Geometry check sheet. Reference: the model listing, model coordinates, mm. A direction names the side the tool comes from. Round coordinates to 2 decimals unless told otherwise and drop trailing zeros. Order: outer loops, then holes, each group sorted by start corner. A loop starts at its lowest first (then second) coordinate and runs counter-clockwise, first axis right, second up.
(1) Set-up check for faces 4 (the face through (11, 0, 12.7)), 5 (the face through (-8, -7, 7.62)): record each of +Z, -Z, +X, -X, +Y, -Y from which the full face is reachable in a straight line by a thin tool's end or side.
(2) Draft check along Y on faces 1 (the face through (-3.472, 26.443, 7.549)), 2 (the face through (13, -24, 2.54)), 3 (the face through (10.902, 3.433, 3.757)). Enter one of: pulls with the +Y half, pulls with the -Y half, needs draft (parallel to the pull), parting line crosses it, or undercut.
(3) Cross-section at A-A on y = 0. Enter the section's corners in (x, z), and give its area (3 significant figures).
(4) Cross-section at C-C on z = 11.25. Enter the section's corners in (x, y).
(5) Cross-section at D-D on x = 21. Enter the section's corners in (y, z).
(6) Thickness scan on L1, parallel to Y at x = 0, z = 3; L2, parallel to Y at x = 0, z = 2.5; L3, parallel to X at y = 0, z = 10.2. Record the ranges inside material, lowest first.
(7) Gauge pin test, flat ends, axial feed: P1, Ø5, axis at y = -22, z = 2.5, coming from the -X side; P2, Ø17.5, axis at x = -1, y = -4, coming from the +Z side; P3, Ø3, axis at y = -11, z = 6, coming from the +X side; P4, Ø20.5, axis at x = 0, y = 0, coming from the -Z side. Record the tip position at first contact, or that the pin passes through.
from build123d import *

# Parameters (mm, degrees)
F0_R     = 29.21
F1_DEPTH = 2.54
F2_R     = 26.67
F3_DEPTH = 12.7
F4_R     = 10.16
F5_DEPTH = 12.701
F6_R     = 11.43
F7_DEPTH = 7.62


with BuildPart() as f1:
    # F0 (on Top) → F1 (new body)
    with BuildSketch(Plane.XY):
        Circle(F0_R)
    extrude(amount=F1_DEPTH)

    # F2 (on Top) → F3 (join)
    with BuildSketch(Plane.XY):
        Circle(F2_R)
    extrude(amount=F3_DEPTH)

    # F4 (on Top) → F5 (cut, through all)
    with BuildSketch(Plane.XY):
        Circle(F4_R)
    extrude(amount=F5_DEPTH, mode=Mode.SUBTRACT)

    # F6 (on Top) → F7 (cut)
    with BuildSketch(Plane.XY):
        Circle(F6_R)
    extrude(amount=F7_DEPTH, mode=Mode.SUBTRACT)


solid = f1.part
Found:
1. face 4: +Z, +X, -X, +Y, -Y
1. face 5: -Z
2. face 1: parting line crosses it
2. face 2: needs draft
2. face 3: undercut
3. outline: (-29.21, 0) - (-11.43, 0) - (-11.43, 7.62) - (-10.16, 7.62) - (-10.16, 12.7) - (-26.67, 12.7) - (-26.67, 2.54) - (-29.21, 2.54) - close; (10.16, 7.62) - (11.43, 7.62) - (11.43, 0) - (29.21, 0) - (29.21, 2.54) - (26.67, 2.54) - (26.67, 12.7) - (10.16, 12.7) - close
3. area: 413 mm2
4. outline: circle Ø53.34 at (0, 0); hole circle Ø20.32 at (0, 0)
5. outline: (-20.3, 0) - (20.3, 0) - (20.3, 2.54) - (16.44, 2.54) - (16.44, 12.7) - (-16.44, 12.7) - (-16.44, 2.54) - (-20.3, 2.54) - close
6. L1: y = -26.67 to -11.43, 11.43 to 26.67
6. L2: y = -29.21 to -11.43, 11.43 to 29.21
6. L3: x = -26.67 to -10.16, 10.16 to 26.67
7. P1: stops at x = -21.75
7. P2: stops at z = 12.7
7. P3: stops at x = 24.92
7. P4: stops at z = 7.62
